from build123d import *

# Parameters (mm, degrees)
SKETCH1_R           = 3
BOSS_EXTRUDE3_DEPTH = 6
SCALE1_SCALE        = 0.5


with BuildPart() as part:
    # Sketch1 → Boss-Extrude3 (new body)
    with BuildSketch(Plane.XY):
        with BuildLine():
            Line((236.346486318, 61.328001261), (233.557157529, 14.05846688))
            ThreePointArc((233.557157529, 14.05846688), (234.631574503, 11.576933684), (237.266269116, 10.968030468))
            Line((237.266269116, 10.968030468), (254.377513225, 21.340067299))
            ThreePointArc((254.377513225, 21.340067299), (278.773329443, 31.985318101), (305.113217886, 35.817744276))
            ThreePointArc((305.113217886, 35.817744276), (308.442395565, 35.909839099), (311.76666015, 36.112744111))
            Line((311.76666015, 36.112744111), (648.006438707, 46.528011178))
            Line((648.006438707, 46.528011178), (648.006438707, 51.498330229))
            Line((648.006438707, 51.498330229), (644.232143491, 57.724965154))
            Line((644.232143491, 57.724965154), (413.007588136, 60.346556463))
            ThreePointArc((413.007588136, 60.346556463), (404.387645707, 60.630259841), (395.787949399, 61.285331218))
            Line((395.787949399, 61.285331218), (254.377513225, 75.129575697))
            ThreePointArc((254.377513225, 75.129575697), (242.203210075, 72.35558012), (236.346486318, 61.328001261))
        make_face()
        with Locations((250.480867538, 65.373411048)):
            Circle(SKETCH1_R, mode=Mode.SUBTRACT)
        with Locations((247.123521652, 25.373411048)):
            Circle(SKETCH1_R, mode=Mode.SUBTRACT)
    extrude(amount=-BOSS_EXTRUDE3_DEPTH)


with BuildPart() as part_1:
    # Scale1: scaled about (389.049818366, 50.358874463, -3)
    add(part.part.scale(SCALE1_SCALE).moved(Location((194.524909183, 25.179437231, -1.5))))


solid = part_1.part
Part model, mm, in its own coordinate system. Give positions to 0.01 mm unless a question says otherwise; leave off trailing zeros. Write each loop counter-clockwise with the first axis right and the second up, starting at its lowest first coordinate (ties: lowest second). Pieces come first, ordered by that corner, then holes.
1) Probe L1, parallel to X at y = 39, z = -2.8; L2, parallel to X at y = 37, z = -1.8; L3, parallel to Y at x = 402.5, z = -3.65. List the from-to ranges inside material, lowest first.
Resolved:
L1: x = 311.7 to 317.1, 319.07 to 327.82
L2: x = 311.59 to 316.86, 319.31 to 323.71
L3: y = 44.85 to 55.34
2) Pin check, flat tips, straight feed: pin 1 (2.5 mm diameter, centred on x = 319.77, y = 57.87, fed in from -Z); pin 2 (1 mm diameter, centred on y = 34.5, z = -3, fed in from -X). Stop position of each tip, or through.
Resolved:
pin 1: passes through
pin 2: stops at x = 311.41
3) Cut at C-C on x = 389. Write the cut outline in (y, z).
Resolved:
outline: (44.43, -4.5) - (56.16, -4.5) - (56.16, -1.5) - (44.43, -1.5) - close
4) Cut at A-A on z = -2.3. Write the cut outline in (x, y).
Resolved:
outline: (311.3, 32.21) arc R1.5 ccw to (313.16, 30.66) - (321.71, 35.85) arc R50 cw to (347.08, 43.09) arc R50 ccw to (350.41, 43.24) - (518.53, 48.44) - (518.53, 50.93) - (516.64, 54.04) - (401.03, 55.35) arc R100 cw to (392.42, 55.82) - (321.71, 62.74) arc R7.5 ccw to (312.7, 55.84) - close; hole circle Ø3 at (318.09, 37.87); hole circle Ø3 at (319.77, 57.87)
5) Cut at B-B on x = 363. Write the cut outline in (y, z).
Resolved:
outline: (43.63, -4.5) - (58.7, -4.5) - (58.7, -1.5) - (43.63, -1.5) - close
